Part print with two shaded views. Sizes in mm from the minimum x, y, z corner. A direction names the side the tool comes from. Give positions to 0.01 mm unless a question says otherwise; leave off trailing zeros. Write each loop counter-clockwise with the first axis right and the second up, starting at its lowest first coordinate (ties: lowest second). Pieces come first, ordered by that corner, then holes. Notation, with made-up numbers: (-18.5, -33.75) -> (9.5, -33.75) arc R19 cw to (9.5, -1.75) -> close; hole circle Ø1 at (-12, -4.75). An arc over 180 degrees is marked (long way). Answer in a Markdown table with one row per item. Add a question column.
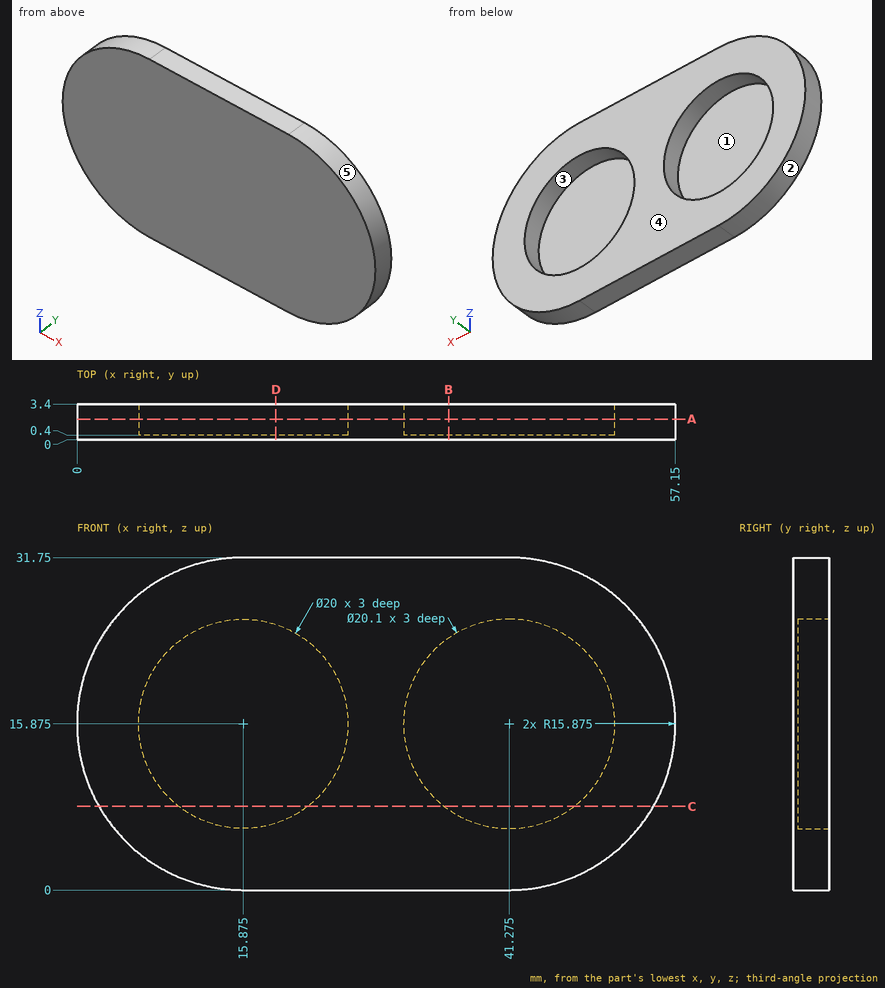
Item 1: Slice it at D-D, the plane x = 19. List the corners of the cut face in (y, z).
Item 2: Drop flat-ended pins along their axis: pin 1 Ø2 at (y, z) = (3, 8.5) entering from -X; pin 2 Ø16 at (x, z) = (41.275, 15.875) entering from +Y; pin 3 Ø1.5 at (x, z) = (49, 8.5) entering from -Y; pin 4 Ø1.5 at (y, z) = (2, 11.5) entering from -X. Give the stop position or say it passes through.
Item 3: Which spindle directions (+Z, -Z, +X, -X, +Y, -Y) get a long thin tool onto all of the face, cutting with end or side? Do the marked faces 1 and 2. Say none if no direction does.
Item 4: Slice it at C-C, the plane z = 8. List the corners of the cut face in (x, y), then the cut area to 3 significant figures.
Item 5: Slice it at B-B, the plane x = 35.5. List the corners of the cut face in (y, z), then the cut area to 3 significant figures.
Item 6: Mould opens along Z. For the marked faces 3, 4 and 5 say: released by +Z, released by -Z, zero draft, split by the parting line, or undercut.
Item 7: Probe L1, parallel to X at y = 1.05, z = 16; L2, parallel to X at y = 0.6, z = 22.5; L3, parallel to Z at x = 41.5, y = 0.9. List the from-to ranges inside material, lowest first. Write a range as from..to.
Item 8: Slice it at A-A, the plane y = 1.95. List the corners of the cut face in (x, z) (3 decimals).
Answer key:
| question | item | result |
|---|---|---|
| 1 | outline | (0, 0) -> (3.4, 0) -> (3.4, 6.38) -> (0.4, 6.38) -> (0.4, 25.37) -> (3.4, 25.37) -> (3.4, 31.75) -> (0, 31.75) -> close |
| 2 | pin 1 | stops at x = 1.34 |
| 2 | pin 2 | stops at y = 0.4 |
| 2 | pin 3 | stops at y = 0 |
| 2 | pin 4 | stops at x = 0.42 |
| 3 | face 1 | +Y |
| 3 | face 2 | -X, +Y, -Y |
| 4 | outline | (2.09, 0) -> (55.06, 0) -> (55.06, 3.4) -> (47.52, 3.4) -> (47.52, 0.4) -> (35.03, 0.4) -> (35.03, 3.4) -> (22.04, 3.4) -> (22.04, 0.4) -> (9.71, 0.4) -> (9.71, 3.4) -> (2.09, 3.4) -> close |
| 4 | area | 106 mm² |
| 5 | outline | (0, 0) -> (3.4, 0) -> (3.4, 7.65) -> (0.4, 7.65) -> (0.4, 24.1) -> (3.4, 24.1) -> (3.4, 31.75) -> (0, 31.75) -> close |
| 5 | area | 58.6 mm² |
| 6 | face 3 | undercut |
| 6 | face 4 | zero draft |
| 6 | face 5 | split by the parting line |
| 7 | L1 | x = 0..5.88, 25.87..31.23, 51.32..57.15 |
| 7 | L2 | x = 1.45..8.38, 23.37..33.72, 48.83..55.7 |
| 7 | L3 | z = 0..5.83, 25.92..31.75 |
| 8 | outline | (15.875, 0) -> (41.275, 0) arc R15.875 ccw to (41.275, 31.75) -> (15.875, 31.75) arc R15.875 ccw to start; hole circle Ø20 at (15.875, 15.875); hole circle Ø20.1 at (41.275, 15.875) |
